```python
from build123d import *

# Parameters (mm, degrees)
F0_W     = 25.4
F0_H     = 31.75
F1_DEPTH = 38.1
F3_DEPTH = 25.401


with BuildPart() as f1:
    # F0 (on Front) → F1 (new body)
    with BuildSketch(Plane.XZ):
        with Locations((-49.920441, 31.029846)):
            Rectangle(F0_W, F0_H)
    extrude(amount=F1_DEPTH)

    # F2 (on face) → F3 (cut, through all)
    with BuildSketch(Plane(origin=(-62.620441, 0, 0), x_dir=(0, -1, 0), z_dir=(-1, 0, 0))):
        Polygon((38.1, 46.904846), (12.7, 46.904846), (25.028251, 27.854846), (38.1, 27.854846), align=None)
    extrude(amount=-F3_DEPTH, mode=Mode.SUBTRACT)


solid = f1.part
```
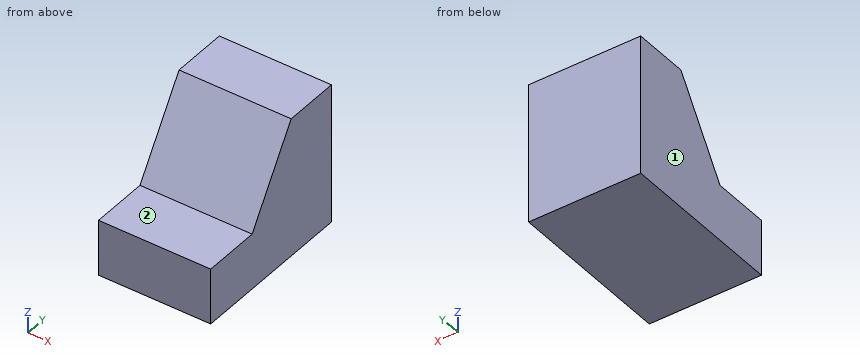
CAD build for the part. Positions are in the model's coordinates, mm. Face numbers are marked on the shaded views. A direction names the side the tool comes from. Give positions to 0.01 mm unless a question says otherwise; leave off trailing zeros. Loops run counter-clockwise (first coordinate to the right, second up) from the corner with the lowest first, then second, coordinate; pieces in that order, holes last. Notation, with made-up numbers: (54.25, 45) -> (60.25, 45) arc R19 cw to (60.25, 65) -> close; hole circle Ø11 at (13.5, -26.5). An arc over 180 degrees is marked (long way). Use a Markdown table: item, result.
1. Which spindle directions (+Z, -Z, +X, -X, +Y, -Y) get a long thin tool onto all of the face, cutting with end or side? Do the marked faces 1 and 2. Say none if no direction does.
Check result:
| item | result |
|---|---|
| face 1 | +Z, -Z, -X, +Y, -Y |
| face 2 | +Z, +X, -X, -Y |
2. Slice it at B-B (y = -28.5). List the corners of the cut face in (x, z).
Check result:
| item | result |
|---|---|
| outline | (-62.62, 15.15) -> (-37.22, 15.15) -> (-37.22, 27.85) -> (-62.62, 27.85) -> close |
3. Slice it at C-C (z = 42). List the corners of the cut face in (x, y), plus the area to 3 significant figures.
Check result:
| item | result |
|---|---|
| outline | (-62.62, -15.87) -> (-37.22, -15.87) -> (-37.22, 0) -> (-62.62, 0) -> close |
| area | 403 mm^2 |
4. Flat gauge pins, fed straight in: pin 1 (1.5 mm diameter, centred on x = -48.5, y = -27.5, fed in from +Z); pin 2 (8 mm diameter, centred on x = -45.5, z = 40, fed in from -Y); pin 3 (8 mm diameter, centred on x = -41.5, y = -17.5, fed in from +Z). Where does each tip first touch, or does it go through?
Check result:
| item | result |
|---|---|
| pin 1 | stops at z = 27.85 |
| pin 2 | stops at y = -19.76 |
| pin 3 | stops at z = 45.67 |
5. Wall check: L1, parallel to Z at x = -60.5, y = -35.5; L2, parallel to Y at x = -45.75, z = 33; L3, parallel to Z at x = -47.5, y = -19.5. Give the ranges that are in metal, low to high. Write a range as [from, to].
Check result:
| item | result |
|---|---|
| L1 | z = [15.15, 27.85] |
| L2 | y = [-21.7, 0] |
| L3 | z = [15.15, 36.4] |
6. Slice it at A-A (x = -44.75). List the corners of the cut face in (y, z).
Check result:
| item | result |
|---|---|
| outline | (-38.1, 15.15) -> (0, 15.15) -> (0, 46.9) -> (-12.7, 46.9) -> (-25.03, 27.85) -> (-38.1, 27.85) -> close |
